```python
from build123d import *

# Parameters (mm, degrees)
SKETCH1_R               = 7
BOSS_EXTRUDE1_DEPTH     = 15
SKETCH2_R               = 8
BOSS_EXTRUDE2_DEPTH     = 15
CUT_EXTRUDE1_DEPTH      = 35.917798754
CUT_EXTRUDE1_DEPTH_BACK = 35.917798754
SKETCH3_R               = 2.5


with BuildPart() as part:
    # Sketch1 → Boss-Extrude1 (new body)
    with BuildSketch(Plane(origin=(0, 0, 0), x_dir=(1, 0, 0), z_dir=(0, 1, 0))):
        with Locations(Location((0, 0, 0), (0, 0, 270))):
            Circle(SKETCH1_R)
    extrude(amount=BOSS_EXTRUDE1_DEPTH)

    # Sketch2 → Boss-Extrude2 (add)
    with BuildSketch(Plane(origin=(0, 15, 0), x_dir=(1, 0, 0), z_dir=(0, 1, 0))):
        with Locations(Location((0, 0, 0), (0, 0, 270))):
            Circle(SKETCH2_R)
    extrude(amount=BOSS_EXTRUDE2_DEPTH)

    # Sketch4 → Revolve1 (revolve)
    with BuildSketch(Plane.XY):
        with BuildLine():
            Line((0, 33), (0, 30))
            Line((0, 30), (8, 30))
            ThreePointArc((8, 30), (4.336527008, 32.397405356), (0, 33))
        make_face()
    revolve(axis=Axis((0, 33, 0), (0, -1, 0)))

    # Sketch3 → Cut-Extrude1 (cut, two sides: drawn at the far end of the back side and taken through both)
    with BuildSketch(Plane(origin=(0, 0, 0), x_dir=(0, 0, -1), z_dir=(1, 0, 0)).offset(-CUT_EXTRUDE1_DEPTH_BACK)):
        with Locations((0, 25)):
            Circle(SKETCH3_R)
    extrude(amount=CUT_EXTRUDE1_DEPTH + CUT_EXTRUDE1_DEPTH_BACK, mode=Mode.SUBTRACT)


solid = part.part
```
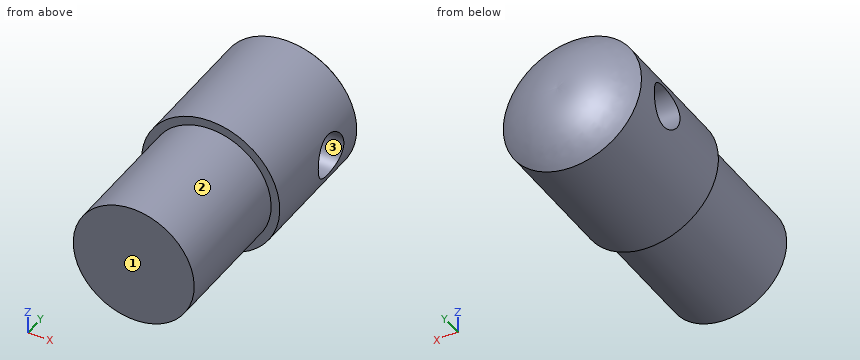
Check sheet for the modelled part. Datum: model origin and axes. Units: mm. Face numbers are marked on the shaded views. Give positions to 0.01 mm unless a question says otherwise; leave off trailing zeros. Write each loop counter-clockwise with the first axis right and the second up, starting at its lowest first coordinate (ties: lowest second). Pieces come first, ordered by that corner, then holes.
Item 1: Cross-section at C-C (y = 11.5). Enter the section's corners in (x, z).
Item 2: Cross-section at B-B (y = 25). Enter the section's corners in (x, z).
Item 3: Draft check along Y on the marked faces 1, 2 and 3. Enter one of: released by +Y, released by -Y, zero draft, split by the parting line, or undercut.
Item 4: Gauge pin test, flat ends, axial feed: pin 1 (1 mm diameter, centred on y = 29, z = 2, fed in from -X); pin 2 (4 mm diameter, centred on y = 13.5, z = 5, fed in from -X); pin 3 (6 mm diameter, centred on x = 5, y = 28.5, fed in from -Z). Record the tip position at first contact, or that the pin passes through.
Item 5: Scan lines: L1, parallel to Y at x = -2.75, z = 0; L2, parallel to Z at x = -4.5, y = 25; L3, parallel to Z at x = -3.5, y = 25. Record each from-to range of solid material in increasing order.
Item 6: Cross-section at A-A (y = 16). Enter the section's corners in (x, z).
Report:
1. outline: circle Ø14 at (0, 0)
2. outline: (-7.6, -2.5) arc R8 ccw to (7.6, -2.5) - close; (-7.6, 2.5) - (7.6, 2.5) arc R8 ccw to start
3. face 1: released by -Y
3. face 2: zero draft
3. face 3: undercut
4. pin 1: stops at x = -7.86
4. pin 2: stops at x = -7.1
4. pin 3: stops at z = -7.75
5. L1: y = 0 to 22.5, 27.5 to 32.85
5. L2: z = -6.61 to -2.5, 2.5 to 6.61
5. L3: z = -7.19 to -2.5, 2.5 to 7.19
6. outline: circle Ø16 at (0, 0)
